Could you check a few things on this model? Use its own coordinates, in mm. Face numbers are marked on the shaded views. A direction names the side the tool comes from. Coordinates: 2 decimals unless noted, no trailing zeros. Write each loop counter-clockwise with the first axis right and the second up, starting at its lowest first coordinate (ties: lowest second). Pieces come first, ordered by that corner, then holes. Notation, with made-up numbers: (44, -1) - (87, -1) arc R21 ccw to (87, 11) - close; hole circle Ø6 at (56, 79). An arc over 180 degrees is marked (long way). Answer as a JSON object with one key per item and string values. Group by question number.
1) If we section it at A-A (y = -4.5): Write out the boundary of the cut face in (x, z).
2) We'd pull the mould along X, two halves only. Please class the marked faces 4, 5 and 6: released by +X, released by -X, zero draft, split by the parting line, or undercut.
3) If we section it at B-B (x = 0): Write out the boundary of the cut face in (y, z), plus the area to 3 significant figures.
4) If we section it at D-D (x = -34): Write out the boundary of the cut face in (y, z).
5) On a 3-axis mill with a long thin cutter (end or side, diameter ignored), from which of +Z, -Z, +X, -X, +Y, -Y can I reach the whole of each face in a straight line? I mean the marked faces 1, 2 and 3. Say none if no direction works.
6) Please list where these lines run through material, in increasing order: line 1 along Y through (x, z) = (3, 12); line 2 along Z through (x, y) = (0, -12); line 3 along X through (y, z) = (2.5, -2).
7) Will these pins go through, and if not, where does the flat tip stop? pin 1 Ø12 at (x, z) = (-32, 5) entering from +Y; pin 2 Ø1.5 at (y, z) = (-5.5, -4.5) entering from -X; pin 3 Ø10 at (x, z) = (-33.5, 2.5) entering from +Y.
8) If we section it at C-C (y = 14.5): Write out the boundary of the cut face in (x, z).
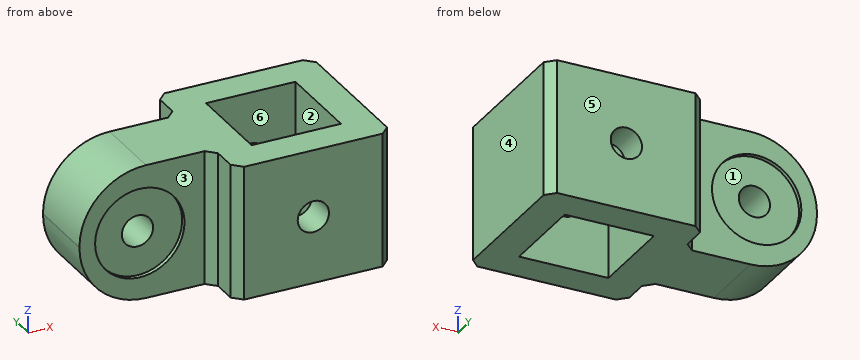
```python
from build123d import *

# Parameters (mm, degrees)
SKETCH_W          = 20
SKETCH_H          = 20
PAD_DEPTH         = 15
SKETCH002_R       = 3.5
POCKET_DEPTH      = 17.501
POCKET_DEPTH_BACK = -17.501
SKETCH001_R       = 10
POCKET001_DEPTH   = 1
SKETCH003_R       = 10
POCKET002_DEPTH   = 1
FILLET_R          = 14.9
CHAMFER_SIZE      = 2


with BuildPart() as part:
    # Sketch → Pad (new body, symmetric)
    with BuildSketch(Plane.XY):
        Polygon((17.5, 17.5), (17.5, -17.5), (-17.5, -17.5), (-17.5, -8), (-47.5, -8), (-47.5, 8), (-17.5, 8), (-17.5, 17.5), align=None)
        Rectangle(SKETCH_W, SKETCH_H, mode=Mode.SUBTRACT)
    extrude(amount=PAD_DEPTH, both=True)

    # Sketch002 → Pocket (cut, two sides)
    with BuildSketch(Plane(origin=(0, 0, 0), x_dir=(-1, 0, 0), z_dir=(0, 1, 0))) as pocket_sk:
        with Locations((34, 0)):
            Circle(SKETCH002_R)
        Circle(SKETCH002_R)
    extrude(amount=-POCKET_DEPTH, mode=Mode.SUBTRACT)
    extrude(pocket_sk.sketch, amount=-POCKET_DEPTH_BACK, mode=Mode.SUBTRACT)

    # Sketch001 (on Face6 of Pad) → Pocket001 (cut)
    with BuildSketch(Plane(origin=(0, 8, 0), x_dir=(-1, 0, 0), z_dir=(0, 1, 0))):
        with Locations((34, 0)):
            Circle(SKETCH001_R)
    extrude(amount=-POCKET001_DEPTH, mode=Mode.SUBTRACT)

    # Sketch003 (on Face4 of Pad) → Pocket002 (cut)
    with BuildSketch(Plane(origin=(0, -8, 0), x_dir=(-1, 0, 0), z_dir=(0, 1, 0))):
        with Locations((34, 0)):
            Circle(SKETCH003_R)
    extrude(amount=POCKET002_DEPTH, mode=Mode.SUBTRACT)

    # Fillet
    fillet_edges = [part.edges().sort_by_distance(p)[0] for p in [
        (-47.5, 0, 15),
        (-47.5, 0, -15),
    ]]
    fillet(fillet_edges, radius=FILLET_R)

    # Chamfer
    chamfer_edges = [part.edges().sort_by_distance(p)[0] for p in [
        (17.5, -17.5, 0),
        (-17.5, -17.5, 0),
        (-17.5, -8, 0),
        (-17.5, 8, 0),
        (17.5, 17.5, 0),
        (-17.5, 17.5, 0),
    ]]
    chamfer(chamfer_edges, length=CHAMFER_SIZE)


solid = part.part
```
Here are the results:
{
 "1": {"outline": "(-47.5, -0.1) arc R14.9 ccw to (-32.6, -15) - (-10, -15) - (-10, 15) - (-32.6, 15) arc R14.9 ccw to (-47.5, 0.1) - close; (10, -15) - (17.5, -15) - (17.5, 15) - (10, 15) - close; hole circle Ø7 at (-34, 0)"},
 "2": {"face 4": "released by +X", "face 5": "zero draft", "face 6": "undercut"},
 "3": {"outline": "(-17.5, -15) - (-10, -15) - (-10, -3.5) - (-17.5, -3.5) - close; (-17.5, 3.5) - (-10, 3.5) - (-10, 15) - (-17.5, 15) - close; (10, -15) - (17.5, -15) - (17.5, -3.5) - (10, -3.5) - close; (10, 3.5) - (17.5, 3.5) - (17.5, 15) - (10, 15) - close", "area": "345 mm²"},
 "4": {"outline": "(-8, -14.93) - (8, -14.93) - (8, -10) - (7, -10) - (7, -3.5) - (-7, -3.5) - (-7, -10) - (-8, -10) - close; (-8, 10) - (-7, 10) - (-7, 3.5) - (7, 3.5) - (7, 10) - (8, 10) - (8, 14.93) - (-8, 14.93) - close"},
 "5": {"face 1": "+Y", "face 2": "+Z, -Z", "face 3": "+Z, -Z, -X, -Y"},
 "6": {"line 1": "y = -17.5 to -10, 10 to 17.5", "line 2": "z = -15 to -3.5, 3.5 to 15", "line 3": "x = -47.38 to -36.87, -31.13 to -10, 10 to 17.5"},
 "7": {"pin 1": "stops at y = 8", "pin 2": "stops at x = -47.05", "pin 3": "stops at y = 7"},
 "8": {"outline": "(-17.5, -15) - (17.5, -15) - (17.5, 15) - (-17.5, 15) - close; hole circle Ø7 at (0, 0)"}
}
